Autodesk Inventor part; units mm, degrees
ref_plane "Start Plane" through (0, 0, 6.35) normal (0, 0, 1) x (1, 0, 0)
ref_plane "End Plane" through (0, 0, 323.85) normal (0, 0, 1) x (1, 0, 0)
ref_plane "Work Plane5" through (-723.9, -555.6504, 6.35) normal (0, 0, -1) x (-1, 0, 0)
ref_plane "Start Plane" through (0, 0, 6.35) normal (0, 0, 1) x (1, 0, 0)
ref_plane "End Plane" through (0, 0, 323.85) normal (0, 0, 1) x (1, 0, 0)
sketch "Sketch" plane through (0, 0, 0) normal (0, 0, 1) x (1, 0, 0)
  line L0 (-12.7, 12.7) -> (12.7, 12.7)
  line L1 (12.7, 12.7) -> (12.7, -12.7)
  line L2 (12.7, -12.7) -> (-12.7, -12.7)
  line L3 (-12.7, -12.7) -> (-12.7, 12.7)
  line L4 (9.525, 9.525) -> (-9.525, 9.525)
  line L5 (-9.525, 9.525) -> (-9.525, -9.525)
  line L6 (-9.525, -9.525) -> (9.525, -9.525)
  line L7 (9.525, -9.525) -> (9.525, 9.525)
  point P0 (0, 0)
  point P1 (0, 12.7)
  point P2 (-12.7, 0)
  dimension "width" = 25.4
  dimension "d1" = 3.175
extrude "Body" add sketch "Sketch" along normal up to surface (317.5 mm away) from surface at 6.35
sketch "Sketch4" plane through (0, 0, 0) normal (0, 0, 1) x (1, 0, 0)
  line L0 (0, 0) -> (10, 0)
ref_plane "Work Plane4" through (0, 0, 0) normal (0, -1, 0) x (1, 0, 0)
sketch "Sketch5" plane through (0, 0, 0) normal (0, -1, 0) x (1, 0, 0)
  line L0 (-2, 6.35) -> (12, 6.35)
  line L1 (-2, 323.85) -> (12, 323.85)
  dimension "d9" = 317.5
ref_plane "Work Plane5" through (-723.9, -555.6504, 6.35) normal (0, 0, -1) x (-1, 0, 0)
split "Split1" plane through (-723.9, -555.6504, 6.35) removes the side toward (0, 0, -1)
ref_plane "Work Plane6" through (-31.75, 631.7996, 323.85) normal (0, 0, 1) x (1, 0, 0)
split "Split2" plane through (-31.75, 631.7996, 323.85) removes the side toward (0, 0, 1)
equation "\"G_OFFSET_START\" = -6.35"
equation "\"G_OFFSET_END\" = 19.05"
equation "\"d4\" = -G_OFFSET_START"
equation "\"d5\" = length + G_OFFSET_END"
equation "\"G_L\" = 304.8"
properties part number "Square Tube Profile"
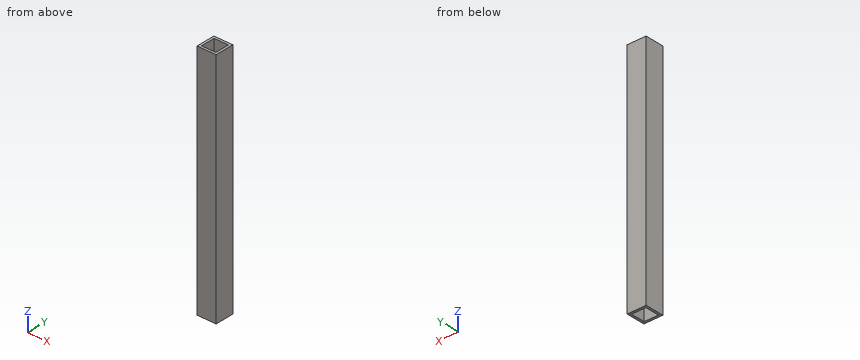
Design review of the part built by this model. Coordinates are the model's own, in mm. Round coordinates to 2 decimals unless told otherwise and drop trailing zeros. Loops run counter-clockwise (first coordinate to the right, second up) from the corner with the lowest first, then second, coordinate; pieces in that order, holes last. Notation, with made-up numbers: (80.25, 65.25) -> (88.25, 65.25) arc R10 cw to (88.25, 69.25) -> close; hole circle Ø1 at (10.25, 76). An arc over 180 degrees is marked (long way). Use one line per item in the form item = value. Start each with the question number.
Q1. Wall thickness on line 1 along X through (y, z) = (1.25, 253.5) (3 decimals): over which ranges is the line inside the solid? List them lowest first. Write a range as [from, to].
Q2. We need section A-A on x = 0.75. Give the boundary of the cut face in (y, z) (3 decimals).
Q3. We need section C-C on z = 304. Give the boundary of the cut face in (x, y) (3 decimals), then the cut area to 3 significant figures.
Q4. For pin 1 Ø6 at (x, y) = (-5, -3.5) entering from -Z, flat-tipped, find the tip position at first contact; note if it passes through.
Calculated:
q1.line_1 = [-12.7, -9.525], [9.525, 12.7]
q2.outline = (-12.7, 6.35) -> (-9.525, 6.35) -> (-9.525, 323.85) -> (-12.7, 323.85) -> close; (9.525, 6.35) -> (12.7, 6.35) -> (12.7, 323.85) -> (9.525, 323.85) -> close
q3.outline = (-12.7, -12.7) -> (12.7, -12.7) -> (12.7, 12.7) -> (-12.7, 12.7) -> close; hole (-9.525, -9.525) -> (9.525, -9.525) -> (9.525, 9.525) -> (-9.525, 9.525) -> close
q3.area = 282 mm²
q4.pin_1 = through
